Autodesk Inventor part; units mm, degrees
ref_plane "YZ Plane" through (0, 0, 0) normal (1, 0, 0) x (0, 1, 0)
ref_plane "XZ Plane" through (0, 0, 0) normal (0, 1, 0) x (-1, 0, 0)
ref_plane "XY Plane" through (0, 0, 0) normal (0, 0, 1) x (1, 0, 0)
sketch "Sketch1" plane through (0, 0, 0) normal (0, 0, 1) x (1, 0, 0)
  circle A0 centre (0, 0) radius 12.12
  circle A1 centre (0, 0) radius 12.62
  arc A2 (10.6143, -11.4595) -> (-10.6143, -11.4595) centre (0, 0) ccw
  line L0 (-12.12, -25) -> (12.12, -25)
  line L1 (12.12, 0) -> (12.12, -25.5944) construction
  line L2 (-12.12, 0) -> (-12.12, -25) construction
  line L3 (-12.12, -25) -> (12.12, -25)
  line L4 (12.12, -25) -> (12.12, -20)
  line L5 (12.12, -20) -> (-12.12, -20)
  line L6 (-12.12, -20) -> (-12.12, -25)
  arc A3 (-12.12, -20) -> (-10.6143, -11.4595) centre (-14.12, -15.2444) ccw
  line L7 (0, 0) -> (0, 15.62) construction
  arc A4 (10.6143, -11.4595) -> (12.12, -20) centre (14.12, -15.2444) ccw
  point P0 (12.12, -25)
  dimension "d0" = 0.5
  dimension "d1" = 3
  dimension "d2" = 25
  dimension "d3" = 5
  dimension "d4" = 2
extrude "Extrusion1" add sketch "Sketch1" against normal blind 25 contours A4 L5 A3 A2 | L4 L0 L6 L5
sketch "Sketch2" plane through (12.12, -25, 0) normal (1, 0, 0) x (0, 0, -1)
  line L0 (0, 0) -> (0, 5)
  line L1 (0, 0) -> (25, 0)
  line L2 (25, 5) -> (25, 0)
  line L3 (0, 5) -> (25, 5)
  point P0 (0, 25)
extrude "Extrusion2" add sketch "Sketch2" along normal blind 10
sketch "Sketch3" plane through (-12.12, -25, 0) normal (-1, 0, 0) x (0, 0, 1)
  line L0 (0, 5) -> (0, 0)
  line L1 (0, 5) -> (-25, 5)
  line L2 (-25, 0) -> (-25, 5)
  line L3 (0, 0) -> (-25, 0)
  point P0 (0, 25)
extrude "Extrusion3" add sketch "Sketch3" along normal blind 10
sketch "Sketch4" plane through (12.12, -20, 0) normal (0, 1, 0) x (1, 0, 0)
  circle A0 centre (7, 12.5) radius 2
  circle A1 centre (-31.24, 12.5) radius 2
  line L0 (7, 12.5) -> (-31.24, 12.5) construction
  line L1 (10, 25) -> (10, 0)
  line L2 (7, 12.5) -> (10, 12.5) construction
  line L3 (10, 0) -> (10, 25)
  line L4 (-34.24, 0) -> (-34.24, 25)
  circle A2 centre (7, 12.5) radius 5
  circle A3 centre (-31.24, 12.5) radius 5
  point P0 (-12.12, 0)
  point P1 (-34.24, 16.5)
  point P2 (-34.24, 8.5)
  point P3 (10, 16.5)
  point P4 (10, 8.5)
  dimension "d11" = 4
  dimension "d12" = 4
  dimension "d13" = 3
  dimension "d14" = 3
  dimension "d17" = 10
  dimension "d18" = 10
extrude "Extrusion4" cut sketch "Sketch4" against normal through all contours A0 | A1
extrude "Extrusion5" add sketch "Sketch4" against normal up to surface (5 mm away) contours A2 L1 | A3 L4 picked at (10.2796, 11.4321) picked at (-35.0103, 13.5108)
fillet "Fillet1" radius 6 4 edges at (22.12, -22.5, -8.5) (22.12, -22.5, -16.5) (-22.12, -22.5, -8.5) (-22.12, -22.5, -16.5)
sketch "Sketch5" plane through (0, 0, 0) normal (0, 0, 1) x (1, 0, 0)
  arc A0 (10.6143, -11.4595) -> (-10.6143, -11.4595) centre (0, 0) ccw
  arc A1 (-12.12, -20) -> (-10.6143, -11.4595) centre (-14.12, -15.2444) ccw
  line L0 (-12.12, -20) -> (-22.12, -20)
  line L1 (-22.12, -25) -> (-22.12, -20)
  line L2 (-22.12, -25) -> (22.12, -25)
  line L3 (22.12, -20) -> (22.12, -25)
  line L4 (12.12, -20) -> (22.12, -20)
  arc A2 (10.6143, -11.4595) -> (12.12, -20) centre (14.12, -15.2444) ccw
  circle A3 centre (0, 0) radius 12.62
  circle A4 centre (0, 0) radius 8.5 construction
  circle A5 centre (0, 8.5) radius 1.5
  line L5 (0, 0) -> (0, 8.5) construction
  circle A6 centre (-8.5, 0) radius 1.5
  circle A7 centre (0, -8.5) radius 1.5
  circle A8 centre (8.5, 0) radius 1.5
  circle A9 centre (0, 0) radius 5
  dimension "d22" = 17
  dimension "d23" = 3
  dimension "d26" = 360
  dimension "d28" = 10
extrude "Extrusion6" add sketch "Sketch5" along normal blind 2 contours A2 L4 L3 L2 L1 L0 A1 A0 | A3
equation "\"d1\" = TB"
equation "\"d5\" = PB"
equation "\"DER\" = 22"
equation "\"HR\" = 7"
equation "\"DIR\" = 8"
equation "\"DEM\" = 4"
equation "\"Dmarc\" = 17.5"
equation "\"Bsm\" = 22.5"
equation "\"Hsm\" = 12"
equation "\"Lsm\" = 21"
equation "\"Dsc\" = 5"
equation "\"RC\" = 7"
equation "\"TB\" = 3"
equation "\"HSE\" = 25"
equation "\"PB\" = 25"
equation "\"LMaSP\" = 46.5"
properties part number "BaseM1"
Geometry check sheet. Reference: the model listing, model coordinates, mm. A direction names the side the tool comes from. Give positions to 0.01 mm unless a question says otherwise; leave off trailing zeros. Loops run counter-clockwise (first coordinate to the right, second up) from the corner with the lowest first, then second, coordinate; pieces in that order, holes last. Notation, with made-up numbers: (65.5, 74) - (98.5, 74) arc R6 ccw to (98.5, 79) - close; hole circle Ø8 at (49, 87.5). An arc over 180 degrees is marked (long way). Use CSV: the item, a comma, the result in double quotes. Start each with the question number.
Q1. Section check B-B, the plane x = 0. Record the cut outline in (y, z).
Q2. Scan lines: probe 1 along X at (y, z) = (-22.55, -12.5); probe 2 along X at (y, z) = (-7, -20.25); probe 3 along X at (y, z) = (7.5, -15). Record each from-to range of solid material in increasing order. Write a range as from..to.
Q3. Section check C-C, the plane y = 0. Record the cut outline in (x, z).
Q4. Release check for a two-part mould opening along Y. For faces 1 (the face through (-17, -20, -11)), 2 (the face through (-22.12, -22, -22)) record: +Y half, -Y half, draft (parallel to the pull), parting line (faces both ways), or undercut.
Q5. Go/stop test with flat-tipped pins: pin 1 Ø11.5 at (x, y) = (0, 0) entering from -Z; pin 2 Ø3.5 at (x, z) = (19.12, -12.5) entering from +Y; pin 3 Ø1.5 at (y, z) = (9, -10) entering from -X; pin 4 Ø5.5 at (y, z) = (-22, -1.5) entering from +X. Record where each tip stops, or that it passes through.
Q6. Access from +Z, -Z, +X, -X, +Y, -Y to the whole of each face (thin tool, end or side, straight path). Record for faces 3 (the face through (-9.052, -16.211, -11.311)), 4 (the face through (22.12, -22, -2)), 5 (the face through (22.12, -22, -22)).
Q7. Section check A-A, the plane x = -19.12. Record the cut outline in (y, z).
Q8. Section check D-D, the plane z = -16.25. Record the cut outline in (x, y).
Findings below:
1,outline,"(-25, -25) - (-12.62, -25) - (-12.62, 0) - (-10, 0) - (-10, 2) - (-25, 2) - close; (-7, 0) - (-5, 0) - (-5, 2) - (-7, 2) - close; (5, 0) - (7, 0) - (7, 2) - (5, 2) - close; (10, 0) - (12.62, 0) - (12.62, -25) - (15.62, -25) - (15.62, 2) - (10, 2) - close"
2,probe 1,"x = -24.12..-21.12, -17.12..17.12, 21.12..24.12"
2,probe 2,"x = -13.96..-10.5, 10.5..13.96"
2,probe 3,"x = -13.7..-10.15, 10.15..13.7"
3,outline,"(-15.62, -25) - (-12.62, -25) - (-12.62, 0) - (-10, 0) - (-10, 2) - (-15.62, 2) - close; (-7, 0) - (-5, 0) - (-5, 2) - (-7, 2) - close; (5, 0) - (7, 0) - (7, 2) - (5, 2) - close; (10, 0) - (12.62, 0) - (12.62, -25) - (15.62, -25) - (15.62, 2) - (10, 2) - close"
4,face 1,"undercut"
4,face 2,"draft"
5,pin 1,"stops at z = 0"
5,pin 2,"passes through"
5,pin 3,"stops at x = -13.26"
5,pin 4,"stops at x = 22.12"
6,face 3,"+Z, -Z, -X"
6,face 4,"+Z, +X, +Y, -Y"
6,face 5,"-Z, +X, +Y, -Y"
7,outline,"(-25, -25) - (-20, -25) - (-20, -14.5) - (-25, -14.5) - close; (-25, -10.5) - (-20, -10.5) - (-20, 2) - (-25, 2) - close"
8,outline,"(-22.7, -25) - (22.7, -25) - (22.7, -20) - (12.12, -20) arc R5.16 cw to (10.61, -11.46) arc R15.62 ccw (long way) to (-10.61, -11.46) arc R5.16 cw to (-12.12, -20) - (-22.7, -20) - close; hole circle Ø25.24 at (0, 0)"
